The model under review builds one solid part; all positions refer to its coordinate system, in mm. A direction names the side the tool comes from. Round coordinates to 2 decimals unless told otherwise and drop trailing zeros. Order: outer loops, then holes, each group sorted by start corner. A loop starts at its lowest first (then second) coordinate and runs counter-clockwise, first axis right, second up.
1) Machinability: for faces 5 (the face through (31.855, -0.2, 154.5)), 6 (the face through (8, 14.5, -2)), 7 (the face through (2, 4.5, -2)), 8 (the face through (41.855, 0.2, -9.5)), 9 (the face through (2, -14.5, -2)), which of the approach directions +Z, -Z, +X, -X, +Y, -Y give a long, thin tool a straight path to every point of the face, cutting with its end or side? Answer none if there is none.
2) Clearance check with flat-ended pins moving along their axes: P1, Ø2, axis at x = 106.5, y = -37, coming from the +Z side; P2, Ø3, axis at y = 0, z = 157.44, coming from the +X side; P3, Ø6.5, axis at y = 0, z = -12.44, coming from the -X side; P4, Ø8, axis at x = 39, z = 155, coming from the -Y side. State where each tip first meets the part, or that it passes through.
3) Mouldability with a two-part tool opening along X and no side actions: class faces 1 (the face through (37, 0, 163.44)), 2 (the face through (-20.39, 0.1, -1.97)), 3 (the face through (31.855, 31.3, 72.9)), 4 (the face through (1, -4.5, -2)) as pulls with the +X half, pulls with the -X half, needs draft (parallel to the pull), parting line crosses it, or undercut.
4) Consider section B-B (y = 0). Give the number of separate pieces and of enclosed holes in the cut face, then the cut area to 3 significant figures.
5) Consider section C-C (x = 3.5). Give the boundary of the cut face in (y, z), then the cut area to 3 significant figures.
6) To check wall thickness, follow L1, parallel to Z at x = 54, y = -27; L2, parallel to Y at x = 38, z = -12; L3, parallel to Y at x = 96, z = 71. State the ranges of each line that lie inside material, in increasing order.
7) Consider section D-D (x = 87). Give the boundary of the cut face in (y, z), then the cut area to 3 significant figures.
8) Consider section A-A (z = 157.44). Give the boundary of the cut face in (x, y), then the cut area to 3 significant figures.
Autodesk Inventor part; units mm, degrees
ref_plane "Płaszczyzna konstrukcyjna1" through (117.8756, 33, 145) normal (0, 0, 1) x (-1, 0, 0)
ref_plane "Płaszczyzna konstrukcyjna4" through (117.8756, 33, 72.5) normal (0, 0, -1) x (-1, 0, 0)
ref_plane "Płaszczyzna konstrukcyjna6" through (0, 0, 72.5) normal (0, 0, 1) x (1, 0, 0)
sketch "Szkic1" plane through (0, 0, 0) normal (0, 0, 1) x (1, 0, 0)
  arc A0 (0, 35) -> (0, -35) centre (0, 0) ccw construction
  line L0 (0, 35) -> (390, 35) construction
  line L1 (0, -35) -> (390, -35) construction
  arc A1 (390, -35) -> (390, 35) centre (390, 0) ccw construction
  circle A2 centre (0, 0) radius 4.5
  circle A3 centre (390, 0) radius 4.5
  line L2 (130, 35) -> (130, 10) construction
  line L3 (260, 35) -> (260, 10) construction
  circle A4 centre (130, 10) radius 25 construction
  circle A5 centre (260, 10) radius 25 construction
  circle A6 centre (130, 10) radius 4.5
  circle A7 centre (260, 10) radius 4.5
  circle A8 centre (0, 0) radius 35 construction
  circle A9 centre (390, 0) radius 35 construction
  line L4 (117.8756, 33) -> (31.8551, 33)
  line L5 (375.6125, 33) -> (272.1244, 33)
  line L6 (247.8756, 33) -> (142.1244, 33)
  line L7 (31.8551, 31) -> (114.6703, 31)
  line L8 (145.3297, 31) -> (244.6703, 31)
  line L9 (275.3297, 31) -> (371.697, 31)
  arc A10 (375.6125, 33) -> (371.697, 31) centre (390, 0) ccw
  arc A11 (117.8756, 33) -> (114.6703, 31) centre (130, 10) ccw
  arc A12 (145.3297, 31) -> (142.1244, 33) centre (130, 10) ccw
  arc A13 (247.8756, 33) -> (244.6703, 31) centre (260, 10) ccw
  arc A14 (275.3297, 31) -> (272.1244, 33) centre (260, 10) ccw
  line L10 (31.8551, 14.5) -> (31.8551, 35) construction
  line L11 (31.8551, 33) -> (31.8551, 31)
  line L12 (260, 10) -> (260, 0)
  line L13 (130, 10) -> (130, 0)
  point P0 (423.5971, -9.8098)
  dimension "d94" = 50
  dimension "d0" = 70
  dimension "d1" = 390
  dimension "d2" = 390
  dimension "d3" = 70
  dimension "d4" = 9
  dimension "d5" = 9
  dimension "d10" = 25
  dimension "d11" = 25
  dimension "d12" = 9
  dimension "d13" = 9
  dimension "d14" = 130
  dimension "d15" = 260
  dimension "d24" = 2
  dimension "d25" = 2
  dimension "d26" = 2
  dimension "d27" = 1
  dimension "d95" = 2
extrude "Wyciągnięcie proste1" add sketch "Szkic1" along normal blind 145 contours A11 L7 L11 L4 | A10 L9 A14 L5 | A13 L8 A12 L6
ref_plane "Płaszczyzna konstrukcyjna1" through (117.8756, 33, 145) normal (0, 0, 1) x (-1, 0, 0)
sketch "Szkic3" plane through (117.8756, 33, 145) normal (0, 0, 1) x (-1, 0, 0)
  circle A0 centre (117.8756, 33) radius 4.5
  arc A1 (133.7659, 28.5) -> (133.7659, 37.5) centre (133.7659, 33) ccw
  arc A2 (98.6659, 37.5) -> (98.6659, 28.5) centre (98.6659, 33) ccw
  line L0 (133.7659, 28.5) -> (98.6659, 28.5)
  line L1 (98.6659, 37.5) -> (133.7659, 37.5)
  line L2 (98.6659, 18.5) -> (133.7659, 18.5)
  arc A3 (133.7659, 18.5) -> (133.7659, 47.5) centre (133.7659, 33) ccw
  line L3 (133.7659, 47.5) -> (98.6659, 47.5)
  line L4 (86.0205, 18.5) -> (86.0205, -2) construction
  line L5 (98.6659, 18.5) -> (86.0205, 18.5)
  line L6 (98.6659, 47.5) -> (86.0205, 47.5)
  line L7 (86.0205, 0) -> (86.0205, 2)
  line L8 (86.0205, 18.5) -> (86.0205, 0)
  line L9 (98.6659, 47.5) -> (98.6659, 81.8113)
  line L10 (98.6659, 81.8113) -> (-234.1244, 81.8113)
  line L11 (-157.4541, 2) -> (-253.8214, 2)
  line L12 (86.0205, 0) -> (86.0205, 2)
  line L13 (-257.7369, 0) -> (-154.2487, 0)
  line L14 (86.0205, 0) -> (-238.0399, 0)
  circle A4 centre (-272.1244, 33) radius 35 construction
  line L15 (-234.1244, 2) -> (-234.1244, 18.5)
  line L16 (-234.1244, 2) -> (-238.0399, 0)
  line L17 (-246.7694, 47.5) -> (-246.7694, 81.8113)
  line L18 (-246.7694, 81.8113) -> (-234.1244, 81.8113)
  line L19 (-303.9795, 47.5) -> (-409.6259, 47.5) construction
  line L20 (-234.1244, 47.5) -> (-246.7694, 47.5)
  line L21 (-234.1244, 18.5) -> (-281.8694, 18.5)
  line L22 (-246.7694, 47.5) -> (-281.8694, 47.5)
  arc A5 (-281.8694, 47.5) -> (-281.8694, 18.5) centre (-281.8694, 33) ccw
  point P0 (-238.0399, 0)
  dimension "d33" = 9
  dimension "d34" = 9
  dimension "d35" = 10
  dimension "d36" = 47.7454
  dimension "d37" = 12.6455
  dimension "d38" = 12.6455
  dimension "d39" = 12.6455
  dimension "d40" = 0
  dimension "d64" = 47.745
  dimension "d93" = 16.5
extrude "Wyciągnięcie proste2" add sketch "Szkic3" along normal blind 4
ref_plane "Płaszczyzna konstrukcyjna4" through (117.8756, 33, 72.5) normal (0, 0, -1) x (-1, 0, 0)
mirror "Odbij2" about plane through (117.8756, 33, 72.5) normal (0, 0, -1) of "Wyciągnięcie proste2"
extrude "Wyciągnięcie proste4" cut sketch "Szkic1" along normal mid plane 10000 contours A6 | A7
sketch "Szkic8" plane through (0, 0, 145) normal (0, 0, 1) x (1, 0, 0)
  line L0 (352, 31) -> (371.697, 31)
  line L1 (352, 31) -> (355.9155, 33)
  line L2 (352, 31) -> (355.9155, 33)
  line L3 (375.6125, 33) -> (355.9155, 33)
  line L4 (355.9155, 33) -> (375.6125, 33)
  arc A0 (375.6125, 33) -> (371.697, 31) centre (390, 0) ccw
  line L5 (375.6125, 33) -> (371.697, 31)
  line L6 (352, 14.5) -> (352, 31)
  line L7 (371.697, 31) -> (352, 31)
  point P0 (0, 0)
  point P1 (352, -48.8113)
ref_plane "Płaszczyzna konstrukcyjna6" through (0, 0, 72.5) normal (0, 0, 1) x (1, 0, 0)
extrude "Wyciągnięcie proste5" cut sketch "Szkic8" along normal mid plane 1000 contours L1 L3 A0 L0
ref_plane "Płaszczyzna konstrukcyjna9" through (117.8756, 33, 149) normal (0, 0, 1) x (1, 0, 0)
sketch "Szkic12" plane through (117.8756, 33, 149) normal (0, 0, 1) x (1, 0, 0)
  line L0 (281.8694, -18.5) -> (234.1244, -18.5)
  arc A0 (281.8694, -47.5) -> (281.8694, -18.5) centre (281.8694, -33) ccw
  line L1 (246.7694, -47.5) -> (281.8694, -47.5)
  line L2 (246.7694, -81.8113) -> (246.7694, -47.5)
  line L3 (234.1244, -2) -> (234.1244, -81.8113)
  line L4 (-98.6659, -81.8113) -> (246.7694, -81.8113)
  point P0 (-117.8756, -33)
extrude "Wyciągnięcie proste7" cut sketch "Szkic12" against normal blind 17
extrude "Wyciągnięcie proste8" cut sketch "Szkic1" against normal blind 17 contours A3
ref_plane "Płaszczyzna konstrukcyjna10" through (117.8756, 33, 149) normal (0, 0, 1) x (1, 0, 0)
sketch "Szkic13" plane through (117.8756, 33, 149) normal (0, 0, 1) x (1, 0, 0)
  line L0 (234.1244, -81.8113) -> (234.1244, -2)
  line L1 (232.1244, -81.8113) -> (232.1244, -2)
  line L2 (234.1244, -2) -> (238.0399, 0)
  line L3 (238.0399, 0) -> (236.0399, 0)
  line L4 (238.0399, 0) -> (-86.0205, 0)
  line L5 (236.0399, 0) -> (232.1244, -2)
  line L6 (238.0399, 0) -> (234.1244, -2)
  line L7 (234.1244, -81.8113) -> (232.1244, -81.8113)
  line L8 (-98.6659, -81.8113) -> (246.7694, -81.8113)
  point P0 (-117.8756, -33)
  dimension "d70" = 2
  dimension "d71" = 2
extrude "Wyciągnięcie proste9" add sketch "Szkic13" along normal blind 17
ref_plane "Płaszczyzna konstrukcyjna11" through (117.8756, 33, 166) normal (0, 0, 1) x (1, 0, 0)
sketch "Szkic14" plane through (117.8756, 33, 166) normal (0, 0, 1) x (1, 0, 0)
  line L0 (232.1244, -81.8113) -> (234.1244, -81.8113)
  line L1 (-98.6659, -81.8113) -> (246.7694, -81.8113)
  line L2 (232.1244, -81.8113) -> (246.7694, -81.8113)
  line L3 (246.7694, -81.8113) -> (246.7694, -47.5)
  line L4 (246.7694, -81.8113) -> (246.7694, -47.5)
  line L5 (246.7694, -47.5) -> (281.8694, -47.5)
  line L6 (246.7694, -47.5) -> (281.8694, -47.5)
  line L7 (281.8694, -18.5) -> (234.1244, -18.5)
  line L8 (234.1244, -81.8113) -> (234.1244, -2)
  arc A0 (281.8694, -47.5) -> (281.8694, -18.5) centre (281.8694, -33) ccw
  circle A1 centre (272.1244, -33) radius 4.5
  line L9 (232.1244, -2) -> (232.1244, -81.8113)
  line L10 (236.0399, 0) -> (232.1244, -2)
  line L11 (238.0399, 0) -> (236.0399, 0)
  line L12 (234.1244, -2) -> (238.0399, 0)
  point P0 (-117.8756, -33)
extrude "Wyciągnięcie proste10" add sketch "Szkic14" along normal blind 4
ref_plane "Płaszczyzna konstrukcyjna12" through (364.645, -48.8113, -4) normal (0, 0, -1) x (-1, 0, 0)
sketch "Szkic15" plane through (364.645, -48.8113, -4) normal (0, 0, -1) x (-1, 0, 0)
  line L0 (332.7899, 63.3113) -> (322.7899, 63.3113)
  line L1 (322.7899, 63.3113) -> (322.7899, 34.3113)
  line L2 (322.7899, 34.3113) -> (332.7899, 34.3113)
  line L3 (332.7899, 34.3113) -> (332.7899, 63.3113)
  point P0 (364.645, 48.8113)
  dimension "d78" = 10
extrude "Wyciągnięcie proste11" add sketch "Szkic15" along normal blind 14.44
ref_plane "Płaszczyzna konstrukcyjna13" through (117.8756, 33, 149) normal (0, 0, 1) x (1, 0, 0)
sketch "Szkic16" plane through (117.8756, 33, 149) normal (0, 0, 1) x (1, 0, 0)
  line L0 (-86.0205, -18.5) -> (-133.7659, -18.5)
  line L1 (-86.0205, -47.5) -> (-76.0205, -47.5)
  line L2 (-86.0205, -18.5) -> (-76.0205, -18.5)
  line L3 (-76.0205, -18.5) -> (-76.0205, -47.5)
  line L4 (-76.0205, -47.5) -> (-86.0205, -47.5)
  line L5 (-86.0205, -47.5) -> (-86.0205, -18.5)
  point P0 (-117.8756, -33)
  point P1 (-86.0205, -47.5)
  dimension "d82" = 10
extrude "Wyciągnięcie proste12" add sketch "Szkic16" along normal blind 14.44
ref_plane "Płaszczyzna konstrukcyjna14" through (31.8551, -14.5, -4) normal (-1, 0, 0) x (0, 0, 1)
sketch "Szkic17" plane through (31.8551, -14.5, -4) normal (-1, 0, 0) x (0, 0, 1)
  line L0 (4, 0) -> (4, 29)
  line L1 (4, 19) -> (-14.44, 19)
  line L2 (-14.44, 29) -> (-14.44, 0)
  line L3 (4, 10) -> (0, 10)
  line L4 (4, 10) -> (-12.44, 10)
  line L5 (4, 18.5) -> (-12.44, 18.5)
  line L6 (-12.44, 18.5) -> (-4.44, 18.5)
  line L7 (-4.44, 18.5) -> (-4.44, 10.5)
  line L8 (-4.44, 10.5) -> (-12.44, 10.5)
  line L9 (-12.44, 10.5) -> (-12.44, 18.5)
  circle A0 centre (-8.44, 14.5) radius 2.5
  point P0 (4, 14.5)
  dimension "d86" = 9
  dimension "d87" = 0.5
  dimension "d88" = 8
  dimension "d89" = 8
  dimension "d90" = 5
extrude "Wyciągnięcie proste13" cut sketch "Szkic17" against normal through all contours A0
mirror "Odbij3" about plane through (117.8756, 33, 72.5) normal (0, 0, -1) of "Wyciągnięcie proste13"
ref_plane "Płaszczyzna konstrukcyjna15" through (364.645, -48.8113, -4) normal (0, 0, -1) x (-1, 0, 0)
sketch "Szkic19" plane through (364.645, -48.8113, -4) normal (0, 0, -1) x (-1, 0, 0)
  circle A0 centre (234.645, 58.8113) radius 4.5
  line L0 (234.645, 58.8113) -> (249.645, 58.8113)
  line L1 (249.645, 93.5676) -> (-84.3243, 93.5676)
  line L2 (-84.3243, 93.5676) -> (-84.3243, -14.4504)
  line L3 (-84.3243, -14.4504) -> (249.645, -14.4504)
  line L4 (249.645, -14.4504) -> (249.645, 93.5676)
  point P0 (364.645, 48.8113)
  dimension "d99" = 15
extrude "Wyciągnięcie proste14" cut sketch "Szkic19" against normal blind 682
ref_plane "Płaszczyzna konstrukcyjna16" through (115, -48.8113, -4) normal (1, 0, 0) x (0, 0, -1)
sketch "Szkic20" plane through (115, -48.8113, -4) normal (1, 0, 0) x (0, 0, -1)
  line L0 (0, 0) -> (-4, 0)
  line L1 (-2, 0) -> (-2, 15)
  line L2 (-153, 81.8113) -> (0, 81.8113)
  line L3 (-2, 81.8113) -> (-2, 66.8113)
  line L4 (-150.5659, 0) -> (-150.5659, 15)
  line L5 (-150.5659, 81.8113) -> (-150.5659, 66.8113)
  line L6 (-153, 81.8113) -> (-153, 63.3113)
  circle A0 centre (-150.5659, 66.8113) radius 1
  circle A1 centre (-150.5659, 15) radius 1
  circle A2 centre (-2, 15) radius 1
  circle A3 centre (-2, 66.8113) radius 1
  point P0 (-4, 48.8113)
  dimension "d103" = 15
  dimension "d104" = 15
  dimension "d105" = 2
  dimension "d106" = 2
  dimension "d107" = 2
  dimension "d108" = 2
extrude "Wyciągnięcie proste15" add sketch "Szkic20" along normal blind 7
ref_plane "Płaszczyzna konstrukcyjna5" through (117.8756, 33, 72.5) normal (0, 0, -1) x (-1, 0, 0)
properties part number "Podstawacz1"
Answer below:
1. face 5: +Z, -X, +Y, -Y
1. face 6: +Z, -Z, -X, +Y
1. face 7: +Z, -Z
1. face 8: -Z, +X, +Y, -Y
1. face 9: +Z, -Z, -X, -Y
2. P1: stops at z = 149
2. P2: passes through
2. P3: stops at x = 31.86
2. P4: stops at y = -14.5
3. face 1: needs draft
3. face 2: undercut
3. face 3: pulls with the -X half
3. face 4: undercut
4. separate pieces: 6
4. enclosed holes: 0
4. area: 999 mm2
5. outline: (-14.5, -4) - (-4.5, -4) - (-4.5, 0) - (-14.5, 0) - close; (-14.5, 145) - (-4.5, 145) - (-4.5, 149) - (-14.5, 149) - close; (4.5, -4) - (14.5, -4) - (14.5, 0) - (4.5, 0) - close; (4.5, 145) - (14.5, 145) - (14.5, 149) - (4.5, 149) - close
5. area: 160 mm2
6. L1: z = -4 to 0, 145 to 149
6. L2: y = -14.5 to -2.46, 2.46 to 14.5
6. L3: y = 31 to 33
7. outline: (-48.81, -4) - (33, -4) - (33, 149) - (-48.81, 149) - (-48.81, 145) - (31, 145) - (31, 0) - (-48.81, 0) - close
7. area: 944 mm2
8. outline: (31.86, -14.5) - (41.86, -14.5) - (41.86, -2.5) - (31.86, -2.5) - close; (31.86, 2.5) - (41.86, 2.5) - (41.86, 14.5) - (31.86, 14.5) - close
8. area: 240 mm2
